Can you work these out from the model? Positions are in its coordinate system, mm. Face numbers are marked on the shaded views. A direction names the side the tool comes from. Round coordinates to 2 decimals unless told otherwise and drop trailing zeros. Write each loop counter-clockwise with the first axis right and the second up, starting at its lowest first coordinate (ties: lowest second). Pieces come first, ordered by that corner, then holes. Notation, with made-up numbers: (-9.75, -29) -> (34.25, -29) arc R17 cw to (34.25, -7) -> close; hole circle Ø9 at (-2, 11). An arc over 180 degrees is marked (long way). Write item = value, one per line. Start each with the question number.
1) Thinking about a two-plate mould opening in X: for the marked faces 4, 5, 6 and 7, which applies, +X half, -X half, draft (parallel to the pull), parting line (faces both ways), or undercut?
2) If I drill on line 1 (X direction, y = -7.25, z = -20.5); line 2 (X direction, y = -4.5, z = -23); line 3 (Z direction, x = 59, y = -13.5), over which ranges is the centre line in solid material (lowest first)?
3) Imagine slicing it at A-A, the plane y = -28.75. State how many separate pieces and enclosed holes the cut face has, then the cut area to 3 significant figures.
4) Imagine slicing it at C-C, the plane x = 60. Please give me the cut outline in (y, z), then the cut area to 3 significant figures.
5) For the marked faces 1, 2 and 3, which set-ups out of +Z, -Z, +X, -X, +Y, -Y let a thin tool reach every point of the face, with its end or its side?
6) Imagine slicing it at D-D, the plane y = -12.5. Please give me the cut outline in (x, z).
7) Imagine slicing it at B-B, the plane x = 20.5. Please give me the cut outline in (y, z).
8) I'm going to push flat-ended pins straight in: pin 1 (1.8 mm diameter, centred on x = 35, y = -23.5, fed in from -Z) (3 decimals); pin 2 (2 mm diameter, centred on y = -10, z = -22, fed in from +X); pin 3 (4.5 mm diameter, centred on x = 28.5, y = -16, fed in from -Z) (3 decimals); pin 4 (3 mm diameter, centred on x = 0, z = 0, fed in from +Y). Where does each tip first touch, or does it pass through?
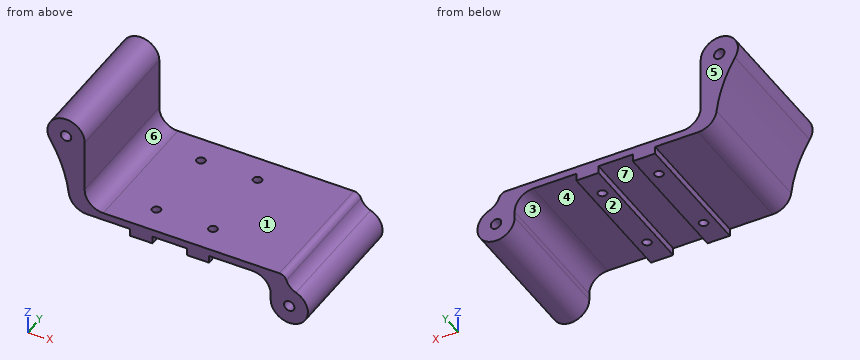
from build123d import *

# Parameters (mm, degrees)
F0_R     = 1.4
F1_DEPTH = 36
F2_R     = 5
F3_W     = 6
F3_H     = 36
F4_DEPTH = 2
F5_R     = 2
F6_R     = 1.15
F7_DEPTH = 4


with BuildPart() as f1:
    # F0 (on Front) → F1 (new body)
    with BuildSketch(Plane.XZ):
        with BuildLine():
            Line((55, -21.085023), (55, -27.809023))
            ThreePointArc((55, -27.809023), (62.833366, -31.928737), (61.788816, -23.139961))
            ThreePointArc((61.788816, -23.139961), (59.764502, -21.545715), (59, -19.085023))
            Line((59, -19.085023), (5, -19.085023))
            Line((5, -19.085023), (5, 0))
            ThreePointArc((5, 0), (-1.368482, 4.809081), (-4.250902, -2.632457))
            ThreePointArc((-4.250902, -2.632457), (-0.338276, -11.492459), (1, -21.085023))
            Line((1, -21.085023), (55, -21.085023))
        make_face()
        with Locations((60, -27.809023)):
            Circle(F0_R, mode=Mode.SUBTRACT)
        Circle(F0_R, mode=Mode.SUBTRACT)
    extrude(amount=F1_DEPTH)

    # F2
    f2_edges = [f1.edges().sort_by_distance(p)[0] for p in [
        (5, -18, -19.085023),
        (1, -18, -21.085023),
        (55, -18, -21.085023),
    ]]
    fillet(f2_edges, radius=F2_R)

    # F3 (on face) → F4 (join)
    with BuildSketch(Plane(origin=(0, 0, -21.085023), x_dir=(1, 0, 0), z_dir=(0, 0, -1))):
        with Locations((20.243325, 18)):
            Rectangle(F3_W, F3_H)
        with Locations((35.443325, 18)):
            Rectangle(F3_W, F3_H)
    extrude(amount=F4_DEPTH)

    # F5
    f5_edges = [f1.edges().sort_by_distance(p)[0] for p in [
        (59, -18, -19.085023),
    ]]
    fillet(f5_edges, radius=F5_R)

    # F6 (on face) → F7 (cut, through all)
    with BuildSketch(Plane(origin=(0, 0, -23.085023), x_dir=(1, 0, 0), z_dir=(0, 0, -1))):
        with Locations((20.243325, 28.75)):
            Circle(F6_R)
        with Locations((35.443325, 28.75)):
            Circle(F6_R)
        with Locations((20.243325, 7.25)):
            Circle(F6_R)
        with Locations((35.443325, 7.25)):
            Circle(F6_R)
    extrude(amount=-F7_DEPTH, mode=Mode.SUBTRACT)


solid = f1.part
Reported:
q1.face_4 = undercut
q1.face_5 = draft
q1.face_6 = +X half
q1.face_7 = undercut
q2.line_1 = 3.34 to 19.09, 21.39 to 34.29, 36.59 to 59.24
q2.line_2 = 17.24 to 23.24, 32.44 to 38.44, 53.93 to 61.46
q2.line_3 = -32.71 to -28.79, -26.83 to -19.99
q3.separate_pieces = 3
q3.enclosed_holes = 2
q3.area = 370 mm²
q4.outline = (-36, -32.81) -> (0, -32.81) -> (0, -29.21) -> (-36, -29.21) -> close; (-36, -26.41) -> (0, -26.41) -> (0, -21.86) -> (-36, -21.86) -> close
q4.area = 293 mm²
q5.face_1 = +Z, +X, +Y, -Y
q5.face_2 = -Z, -X, +Y, -Y
q5.face_3 = -Z, +Y, -Y
q6.outline = (-4.25, -2.63) arc R35.05 cw to (0.73, -16.71) arc R5 ccw to (5.69, -21.09) -> (17.24, -21.09) -> (17.24, -23.09) -> (23.24, -23.09) -> (23.24, -21.09) -> (32.44, -21.09) -> (32.44, -23.09) -> (38.44, -23.09) -> (38.44, -21.09) -> (50, -21.09) arc R5 cw to (55, -26.09) -> (55, -27.81) arc R5 ccw (long way) to (61.79, -23.14) arc R4.34 cw to (59.22, -20.45) arc R2 ccw to (57.32, -19.09) -> (10, -19.09) arc R5 cw to (5, -14.09) -> (5, 0) arc R5 ccw (long way) to start; hole circle Ø2.8 at (0, 0); hole circle Ø2.8 at (60, -27.81)
q7.outline = (-36, -23.09) -> (-29.87, -23.09) -> (-29.87, -19.09) -> (-36, -19.09) -> close; (-27.63, -23.09) -> (-8.37, -23.09) -> (-8.37, -19.09) -> (-27.63, -19.09) -> close; (-6.13, -23.09) -> (0, -23.09) -> (0, -19.09) -> (-6.13, -19.09) -> close
q8.pin_1 = -23.085
q8.pin_2 = 61.46
q8.pin_3 = -21.085
q8.pin_4 = 0
